Read the model definition and answer for the solid it produces. Units are mm, in the model's axes. A direction names the side the tool comes from. Give positions to 0.01 mm unless a question says otherwise; leave off trailing zeros. Loops run counter-clockwise (first coordinate to the right, second up) from the corner with the lowest first, then second, coordinate; pieces in that order, holes last. Notation, with made-up numbers: (15, 47) -> (26, 47) arc R27 ccw to (26, 72) -> close; hole circle Ø6 at (3.25, 44.5). An arc over 180 degrees is marked (long way). One line per item, written item: value. Start each with the question number.
Autodesk Inventor part; units mm, degrees
ref_plane "YZ Plane" through (0, 0, 0) normal (1, 0, 0) x (0, 1, 0)
ref_plane "XZ Plane" through (0, 0, 0) normal (0, 1, 0) x (-1, 0, 0)
ref_plane "XY Plane" through (0, 0, 0) normal (0, 0, 1) x (1, 0, 0)
sketch "Sketch1" plane through (0, 0, 0) normal (0, 0, 1) x (1, 0, 0)
  line L0 (0, 0) -> (0, 38.608)
  line L1 (0, 38.608) -> (73.787, 38.608)
  arc A0 (73.787, 38.608) -> (75.3246, 27.2) centre (97.4163, 35.9853) ccw
  line L2 (0, 0) -> (44.45, 0)
  arc A1 (44.45, 0) -> (75.3246, 27.2) centre (44.45, 31.1228) ccw
  dimension "d1" = 38.608
  dimension "d2" = 73.787
  dimension "d7" = 44.45
extrude "Extrusion1" add sketch "Sketch1" along normal blind 83.693
sketch "Sketch2" plane through (0, 38.608, 0) normal (0, 1, 0) x (1, 0, 0)
  line L0 (0, 0) -> (0, -83.693)
  line L1 (0, 0) -> (73.787, 0)
  line L2 (0, 0) -> (0, -83.693)
  line L3 (73.787, -83.693) -> (0, -83.693)
  line L4 (73.787, 0) -> (73.787, -83.693)
  line L5 (73.787, 0) -> (73.787, -83.693)
  line L6 (73.787, -17.653) -> (60.198, -17.653)
  line L7 (22.352, -17.653) -> (57.023, -17.653)
  line L8 (60.198, -20.828) -> (60.198, -62.865)
  line L9 (57.023, -66.04) -> (22.352, -66.04)
  line L10 (19.177, -62.865) -> (19.177, -20.828)
  arc A0 (22.352, -17.653) -> (19.177, -20.828) centre (22.352, -20.828) ccw
  arc A1 (60.198, -20.828) -> (57.023, -17.653) centre (57.023, -20.828) ccw
  arc A2 (19.177, -62.865) -> (22.352, -66.04) centre (22.352, -62.865) ccw
  arc A3 (57.023, -66.04) -> (60.198, -62.865) centre (57.023, -62.865) ccw
  point P0 (19.177, -17.653)
  point P1 (60.198, -66.04)
  point P2 (19.177, -66.04)
  dimension "d13" = 13.589
  dimension "d14" = 48.387
  dimension "d26" = 41.021
  dimension "d29" = 3.175
extrude "Extrusion2" cut sketch "Sketch2" against normal blind 19.05 contours L7 A1 L8 A3 L9 A2 L10 A0
sketch "Sketch3" plane through (0, 0, 0) normal (-1, 0, 0) x (0, 0, 1)
  line L0 (0, 0) -> (0, 38.608)
  line L1 (0, 0) -> (83.693, 0)
  line L2 (83.693, 38.608) -> (83.693, 0)
  line L3 (0, 38.608) -> (83.693, 38.608)
  line L4 (0, 38.608) -> (83.693, 38.608)
  line L5 (8.9535, 10.1981) -> (8.9535, 28.3591)
  line L6 (12.1285, 7.0231) -> (71.6915, 7.0231)
  line L7 (74.8665, 10.1981) -> (74.8665, 28.3591)
  line L8 (71.6915, 31.5341) -> (12.1285, 31.5341)
  arc A0 (74.8665, 28.3591) -> (71.6915, 31.5341) centre (71.6915, 28.3591) ccw
  arc A1 (12.1285, 31.5341) -> (8.9535, 28.3591) centre (12.1285, 28.3591) ccw
  arc A2 (8.9535, 10.1981) -> (12.1285, 7.0231) centre (12.1285, 10.1981) ccw
  arc A3 (71.6915, 7.0231) -> (74.8665, 10.1981) centre (71.6915, 10.1981) ccw
  point P0 (8.9535, 7.0231)
  point P1 (8.9535, 31.5341)
  point P2 (74.8665, 7.0231)
  point P3 (74.8665, 31.5341)
  dimension "d20" = 24.511
  dimension "d21" = 65.913
  dimension "d28" = 3.175
extrude "Extrusion3" cut sketch "Sketch3" against normal blind 19.05 contours L5 A1 L8 A0 L7 A3 L6 A2
fillet "Fillet2" radius 3.175 8 edges at (36.8935, 38.608, 83.693) (36.8935, 38.608, 0) (73.8549, 32.8095, 83.693) (22.225, 0, 83.693) (65.0236, 7.7699, 83.693) (73.8549, 32.8095, 0) (22.225, 0, 0) (65.0236, 7.7699, 0)
sketch "Sketch4" plane through (0, 0, 83.693) normal (0, 0, 1) x (1, 0, 0)
  circle A0 centre (41.6613, 12.7) radius 3.175
  line L0 (0, 0) -> (44.45, 0)
  dimension "d31" = 6.35
  dimension "d32" = 12.7
extrude "Extrusion4" cut sketch "Sketch4" against normal through all
Item 1: Section D-D, the plane z = 8 is taken. Determine the outline of the cut face in (x, y) (3 decimals).
Item 2: Flat-ended cylindrical pins translate along their axes: pin 1 (3 mm diameter, centred on y = 10.5, z = 34, fed in from -X); pin 2 (5.5 mm diameter, centred on x = 41.66, y = 12.7, fed in from -Z); pin 3 (2 mm diameter, centred on y = 30.5, z = 33, fed in from +X); pin 4 (12 mm diameter, centred on x = 63, z = 65, fed in from -Y). Find the tip coordinate at first contact, or state that the pin passes through.
Item 3: Section A-A, the plane z = 33.5 is taken. Determine the outline of the cut face in (x, y) (3 decimals), plus the area to 3 significant figures.
Item 4: For faces 4 (the cylindrical face through (59.243, 29.216, 65.135)), 5 (the cylindrical face through (9.392, 7.928, 73.912)), 6 (the cylindrical face through (73.866, 32.729, 41.305)), determine the directions among +Z, -Z, +X, -X, +Y, -Y from which every point of the face is accessible in a straight line to the end or side of a thin tool.
Item 5: Consider L1, parallel to Z at x = 12, y = 11; L2, parallel to Z at x = 25.5, y = 25; L3, parallel to Y at x = 16.5, z = 48.5. Determine where each line is inside the solid, lowest interval first. Write a range as [from, to].
Item 6: Section C-C, the plane x = 33.5 is taken. Determine the outline of the cut face in (y, z) (3 decimals).
Item 7: Determine the mould class of faces 1 (the flat face through (36, 20, 83.693)), 2 (the flat face through (60.198, 29, 42)), 3 (the cylindrical face through (65.26, 7.98, 41.31)) for opening direction Z: pulls with the +Z half, pulls with the -Z half, needs draft (parallel to the pull), parting line crosses it, or undercut.
Computed values:
1. outline: (0, 0) -> (44.45, 0) arc R31.123 ccw to (75.325, 27.2) arc R23.775 cw to (73.787, 38.608) -> (0, 38.608) -> close; hole circle Ø6.35 at (41.661, 12.7)
2. pin 1: x = 19.05
2. pin 2: through
2. pin 3: x = 74.54
2. pin 4: y = 2.64
3. outline: (0, 0) -> (44.45, 0) arc R31.123 ccw to (75.325, 27.2) arc R23.775 cw to (73.787, 38.608) -> (60.198, 38.608) -> (60.198, 19.558) -> (19.177, 19.558) -> (19.177, 38.608) -> (0, 38.608) -> (0, 31.534) -> (19.05, 31.534) -> (19.05, 7.023) -> (0, 7.023) -> close; hole circle Ø6.35 at (41.661, 12.7)
3. area: 1,410 mm²
4. face 4: +Y
4. face 5: -X
4. face 6: +Z, -Z, +X
5. L1: [0, 8.95], [74.87, 83.69]
5. L2: [0, 17.65], [66.04, 83.69]
5. L3: [0, 7.02], [31.53, 38.61]
6. outline: (0, 3.175) arc R3.175 ccw to (3.175, 0) -> (35.433, 0) arc R3.175 ccw to (38.608, 3.175) -> (38.608, 17.653) -> (19.558, 17.653) -> (19.558, 66.04) -> (38.608, 66.04) -> (38.608, 80.518) arc R3.175 ccw to (35.433, 83.693) -> (3.175, 83.693) arc R3.175 ccw to (0, 80.518) -> close
7. face 1: pulls with the +Z half
7. face 2: undercut
7. face 3: needs draft
